Study the drawing (mm; zero at the part's minimum x, y, z) and answer. A direction names the side the tool comes from. Round coordinates to 2 decimals unless told otherwise and drop trailing zeros. Write each loop counter-clockwise with the first axis right and the second up, starting at its lowest first coordinate (ties: lowest second). Pieces come first, ordered by that corner, then holes. Notation, with made-up numbers: (7.5, -12) -> (44.5, -12) arc R16 ccw to (44.5, 18) -> close; hole circle Ø2 at (84, 48). An arc over 180 degrees is marked (long way). Return JSON: item names as keys, results as strings.
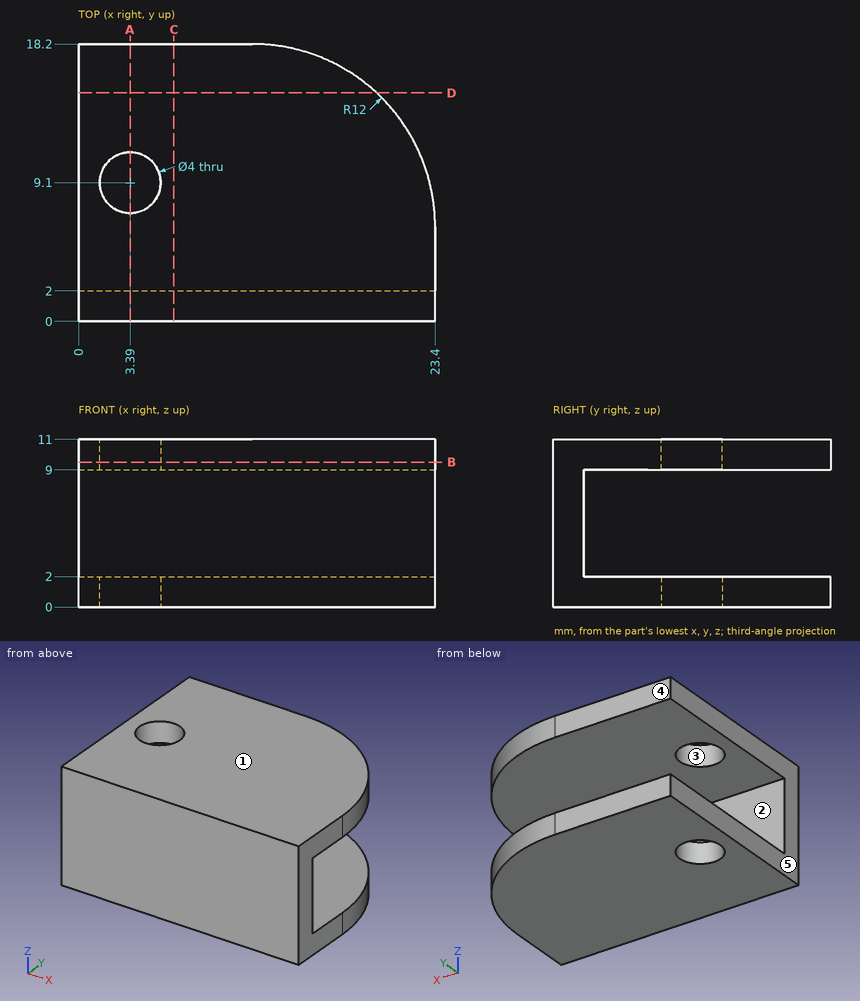
Item 1: Section D-D (y = 15) is taken. Give the vertices of the cut face in (x, z), then the cut area to 3 significant figures.
Worked answers:
{"outline": "(0, 0) -> (19.56, 0) -> (19.56, 2) -> (0, 2) -> close; (0, 9) -> (19.56, 9) -> (19.56, 11) -> (0, 11) -> close", "area": "78.2 mm2"}
Item 2: Flat-ended cylindrical pins translate along their axes: pin 1 (3.5 mm diameter, centred on x = 3.39, y = 9.1, fed in from +Z); pin 2 (3 mm diameter, centred on y = 10, z = 8.5, fed in from +X); pin 3 (5.5 mm diameter, centred on x = 16.5, z = 6, fed in from +Y). Find the tip coordinate at first contact, or state that the pin passes through.
Worked answers:
{"pin 1": "passes through", "pin 2": "stops at x = 23.16", "pin 3": "stops at y = 2"}
Item 3: A tool of negligible diameter and unlimited length cuts with its end or side. For the marked faces 1 and 2, from which of +Z, -Z, +X, -X, +Y, -Y can it reach the whole face along a straight path? Write none if from no direction.
Worked answers:
{"face 1": "+Z, +X, -X, +Y, -Y", "face 2": "+X, -X, +Y"}
Item 4: Section C-C (x = 6.25) is taken. Give the vertices of the cut face in (y, z), then the cut area to 3 significant figures.
Worked answers:
{"outline": "(0, 0) -> (18.2, 0) -> (18.2, 2) -> (2, 2) -> (2, 9) -> (18.2, 9) -> (18.2, 11) -> (0, 11) -> close", "area": "86.8 mm2"}
Item 5: Section B-B (z = 9.5) is taken. Give the vertices of the cut face in (x, y).
Worked answers:
{"outline": "(0, 0) -> (23.4, 0) -> (23.4, 6.2) arc R12 ccw to (11.4, 18.2) -> (0, 18.2) -> close; hole circle Ø4 at (3.39, 9.1)"}
Item 6: Section A-A (x = 3.39) is taken. Give the vertices of the cut face in (y, z).
Worked answers:
{"outline": "(0, 0) -> (7.1, 0) -> (7.1, 2) -> (2, 2) -> (2, 9) -> (7.1, 9) -> (7.1, 11) -> (0, 11) -> close; (11.1, 0) -> (18.2, 0) -> (18.2, 2) -> (11.1, 2) -> close; (11.1, 9) -> (18.2, 9) -> (18.2, 11) -> (11.1, 11) -> close"}
Item 7: Straight lines are drawn through the part: L1, parallel to Z at x = 21.5, y = 11; L2, parallel to Y at x = 3.39, z = 9.75; L3, parallel to Y at x = 13, z = 8.75. For each, find the intervals that lie inside material, in ascending order. Write a range as [from, to].
Worked answers:
{"L1": "z = [0, 2], [9, 11]", "L2": "y = [0, 7.1], [11.1, 18.2]", "L3": "y = [0, 2]"}
Item 8: For a pull along Y with two mould halves and no side action, classify the marked faces 3, 4 and 5 as released by +Y, released by -Y, zero draft, split by the parting line, or undercut.
Worked answers:
{"face 3": "undercut", "face 4": "released by +Y", "face 5": "zero draft"}
